from build123d import *

# Parameters (mm, degrees)
F0_R     = 3.175
F1_DEPTH = 3.048


with BuildPart() as f1:
    # F0 (on Front) → F1 (new body)
    with BuildSketch(Plane.XZ):
        with BuildLine():
            ThreePointArc((-9.525, 114.3), (0, 104.775), (9.525, 114.3))
            ThreePointArc((9.525, 114.3), (0, 123.825), (-9.525, 114.3))
        make_face()
        with Locations((0, 114.3)):
            Circle(F0_R, mode=Mode.SUBTRACT)
        with BuildLine():
            Line((15.7748262685, 58.9305845108), (9.525, 114.3))
            ThreePointArc((9.525, 114.3), (0, 104.775), (-9.525, 114.3))
            Line((-9.525, 114.3), (-15.7748262685, 58.9305845108))
            ThreePointArc((-15.7748262685, 58.9305845108), (0, 73.025), (15.7748262685, 58.9305845108))
        make_face()
        with Locations((-3.175, 93.6752)):
            Circle(F0_R, mode=Mode.SUBTRACT)
        with BuildLine():
            ThreePointArc((15.875, 57.15), (15.8499367824, 58.0417000584), (15.7748262685, 58.9305845108))
            ThreePointArc((15.7748262685, 58.9305845108), (0, 73.025), (-15.7748262685, 58.9305845108))
            ThreePointArc((-15.7748262685, 58.9305845108), (-15.8734077732, 56.9251652464), (-15.7180667333, 54.9233426018))
            ThreePointArc((-15.7180667333, 54.9233426018), (0, 41.275), (15.7180667333, 54.9233426018))
            ThreePointArc((15.7180667333, 54.9233426018), (15.8357180827, 56.0339095893), (15.875, 57.15))
        make_face()
        with Locations((0, 57.15)):
            Circle(F0_R, mode=Mode.SUBTRACT)
        with BuildLine():
            ThreePointArc((15.7180667333, 54.9233426018), (0, 41.275), (-15.7180667333, 54.9233426018))
            Line((-15.7180667333, 54.9233426018), (-7.9375, 0))
            ThreePointArc((-7.9375, 0), (-5.6126600757, 5.6126600757), (0, 7.9375))
            Line((0, 7.9375), (9.0619444624, 7.9375))
            Line((9.0619444624, 7.9375), (15.7180667333, 54.9233426018))
        make_face()
        with BuildLine():
            ThreePointArc((0, 7.9375), (-5.6126600757, 5.6126600757), (-7.9375, 0))
            ThreePointArc((-7.9375, 0), (-5.6126600757, -5.6126600757), (0, -7.9375))
            ThreePointArc((0, -7.9375), (5.6126600757, -5.6126600757), (7.9375, 0))
            ThreePointArc((7.9375, 0), (5.6126600757, 5.6126600757), (0, 7.9375))
        make_face()
        Circle(F0_R, mode=Mode.SUBTRACT)
        with BuildLine():
            Line((44.45, 7.9375), (9.0619444624, 7.9375))
            Line((9.0619444624, 7.9375), (7.9375, 0))
            ThreePointArc((7.9375, 0), (5.6126600757, -5.6126600757), (0, -7.9375))
            Line((0, -7.9375), (44.45, -7.9375))
            ThreePointArc((44.45, -7.9375), (36.5125, 0), (44.45, 7.9375))
        make_face()
        with BuildLine():
            Line((7.9375, 0), (9.0619444624, 7.9375))
            Line((9.0619444624, 7.9375), (0, 7.9375))
            ThreePointArc((0, 7.9375), (5.6126600757, 5.6126600757), (7.9375, 0))
        make_face()
        with BuildLine():
            ThreePointArc((52.3875, 0), (50.0626600757, 5.6126600757), (44.45, 7.9375))
            ThreePointArc((44.45, 7.9375), (36.5125, 0), (44.45, -7.9375))
            ThreePointArc((44.45, -7.9375), (50.0626600757, -5.6126600757), (52.3875, 0))
        make_face()
        with Locations((44.45, 0)):
            Circle(F0_R, mode=Mode.SUBTRACT)
    extrude(amount=F1_DEPTH)


solid = f1.part
Geometry: final body of the model. Coordinates: model frame, mm. A direction names the side the tool comes from. Give positions to 0.01 mm unless a question says otherwise; leave off trailing zeros. Write each loop counter-clockwise with the first axis right and the second up, starting at its lowest first coordinate (ties: lowest second). Pieces come first, ordered by that corner, then holes.
(1) Mould query, pull axis Z, two halves, no side actions, for faces 1 (the flat face through (3, -3.048, 44)), 2 (the flat face through (27, -2, 7.938)), 3 (the flat face through (12.694, -1.503, 86.228)). Classes: released by +Z, released by -Z, zero draft, split by the parting line, or undercut.
(2) Ray query, line 1 (Z direction, x = 32.5, y = -2.4); line 2 (X direction, y = -0.6, z = 96); line 3 (X direction, y = -1.1, z = 85). Return the intervals inside material, ascending.
(3) Cut plane C-C, the plane z = 87. Return loops of the section in (x, y), then the cut area to 3 significant figures.
(4) First-contact query: P1, Ø1, axis at x = 38.5, y = -2, coming from the +Z side. Flat tip, straight axial feed; report the tip coordinate or a pass-through.
(5) Cut plane B-B, the plane x = 36. Return loops of the section in (y, z).
(6) Cut plane A-A, the plane y = -2. Give the number of separate pieces and of enclosed holes in the cut face, then the cut area to 3 significant figures.
(7) Access query for faces 4 (the flat face through (12.343, -1.503, 31.102)), 5 (the cylindrical face through (-15.874, -1.503, 56.953)). Directions: +Z, -Z, +X, -X, +Y, -Y. A direction counts if a zero-diameter tool reaches every point of the face in a straight line with its end or side. Return the directions, or none.
Values follow:
1. face 1: zero draft
1. face 2: undercut
1. face 3: released by +Z
2. line 1: z = -7.94 to 7.94
2. line 2: x = -11.59 to -5.34, -1.01 to 11.59
2. line 3: x = -12.83 to 12.83
3. outline: (-12.61, -3.05) - (12.61, -3.05) - (12.61, 0) - (-12.61, 0) - close
3. area: 76.8 mm2
4. P1: stops at z = 7.94
5. outline: (-3.05, -7.94) - (0, -7.94) - (0, 7.94) - (-3.05, 7.94) - close
6. separate pieces: 1
6. enclosed holes: 5
6. area: 3,600 mm2
7. face 4: +X, +Y, -Y
7. face 5: -X, +Y, -Y
